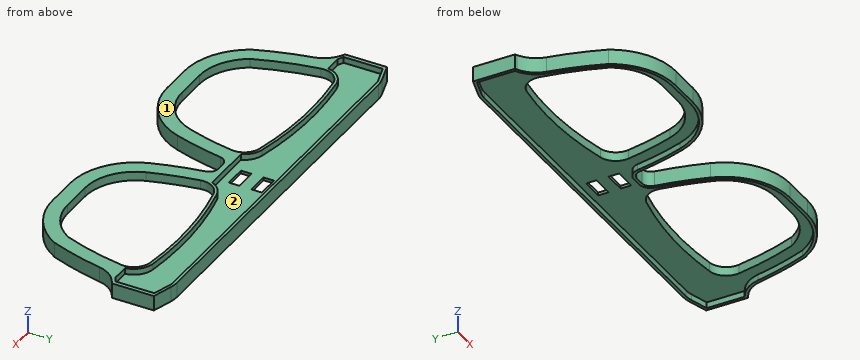
from build123d import *

# Parameters (mm, degrees)
BOSS_EXTRUDE1_DEPTH  = 5
CUT_EXTRUDE1_DEPTH   = 78.98076686
FILLET1_R            = 6
FILLET4_R            = 3
FILLET5_R            = 10
FILLET1_OF_MIRROR2_R = 6
FILLET4_OF_MIRROR2_R = 3
FILLET5_OF_MIRROR2_R = 10
CUT_EXTRUDE2_DEPTH   = 2
SKETCH4_W            = 7.3
SKETCH4_H            = 3.5
CUT_EXTRUDE3_DEPTH   = 78.878110027
CUT_EXTRUDE4_START   = -1
CUT_EXTRUDE4_DEPTH   = 2


with BuildPart() as part:
    # Sketch1 → Boss-Extrude1 (new body)
    with BuildSketch(Plane.XY):
        with BuildLine():
            Line((-70, 16.58258549), (-70, 2.58258549))
            Line((-70, 2.58258549), (-65, -0.035347018))
            ThreePointArc((-65, -0.035347018), (-62.639321295, -11.428715409), (-59.057390955, -22.499009997))
            ThreePointArc((-59.057390955, -22.499009997), (-50.858075368, -30.911196539), (-39.524366721, -34))
            Line((-39.524366721, -34), (-29.119439011, -34))
            ThreePointArc((-29.119439011, -34), (-16.364659062, -29.873537236), (-8.443933007, -19.058075838))
            ThreePointArc((-8.443933007, -19.058075838), (-5.792248942, -9.629238804), (-4, 0))
            Line((-4, 0), (0, 0))
            Line((0, 0), (0, 19))
            Line((0, 19), (-62, 19))
            Line((-62, 19), (-70, 16.58258549))
        make_face()
    boss_extrude1 = extrude(amount=BOSS_EXTRUDE1_DEPTH)

    # Sketch2 → Cut-Extrude1 (cut, through all)
    with BuildSketch(Plane.XY.offset(5)):
        with BuildLine():
            Line((-39.524366721, -29), (-29.119439011, -29))
            ThreePointArc((-29.119439011, -29), (-19.293350153, -25.821035725), (-13.191343035, -17.488968441))
            ThreePointArc((-13.191343035, -17.488968441), (-10.661621804, -8.493805879), (-8.951806424, 0.692541077))
            ThreePointArc((-8.951806424, 0.692541077), (-8.83111114, 2.375291538), (-8.93749946, 4.05900707))
            ThreePointArc((-8.93749946, 4.05900707), (-33.987475013, 7.999161751), (-59.288689209, 6.303681198))
            ThreePointArc((-59.288689209, 6.303681198), (-60.075532666, 3.563074376), (-60.056140486, 0.711816353))
            ThreePointArc((-60.056140486, 0.711816353), (-57.852345066, -9.972645379), (-54.521869403, -20.361214511))
            ThreePointArc((-54.521869403, -20.361214511), (-48.178176596, -26.685865227), (-39.524366721, -29))
        make_face()
    cut_extrude1 = extrude(amount=-CUT_EXTRUDE1_DEPTH, mode=Mode.SUBTRACT)

    # Fillet1
    fillet1_edges = [part.edges().sort_by_distance(p)[0] for p in [
        (-8.93749946, 4.05900707, 2.5),
        (-59.288689209, 6.303681198, 2.5),
    ]]
    fillet(fillet1_edges, radius=FILLET1_R)

    # Fillet4
    fillet4_edges = [part.edges().sort_by_distance(p)[0] for p in [
        (-4, 0, 2.5),
    ]]
    fillet(fillet4_edges, radius=FILLET4_R)

    # Fillet5
    fillet5_edges = [part.edges().sort_by_distance(p)[0] for p in [
        (-65, -0.035347018, 2.5),
        (-62, 19, 2.5),
    ]]
    fillet(fillet5_edges, radius=FILLET5_R)

    # Mirror2: Boss-Extrude1, Cut-Extrude1 across plane
    add(boss_extrude1.mirror(Plane(origin=(0, 19, 5), x_dir=(0, 0, 1), z_dir=(1, 0, 0))))
    add(cut_extrude1.mirror(Plane(origin=(0, 19, 5), x_dir=(0, 0, 1), z_dir=(1, 0, 0))), mode=Mode.SUBTRACT)

    # Fillet1 of Mirror2
    fillet1_of_mirror2_edges = [part.edges().sort_by_distance(p)[0] for p in [
        (8.93749946, 4.05900707, 2.5),
        (59.288689209, 6.303681198, 2.5),
    ]]
    fillet(fillet1_of_mirror2_edges, radius=FILLET1_OF_MIRROR2_R)

    # Fillet4 of Mirror2
    fillet4_of_mirror2_edges = [part.edges().sort_by_distance(p)[0] for p in [
        (4, 0, 2.5),
    ]]
    fillet(fillet4_of_mirror2_edges, radius=FILLET4_OF_MIRROR2_R)

    # Fillet5 of Mirror2
    fillet5_of_mirror2_edges = [part.edges().sort_by_distance(p)[0] for p in [
        (65, -0.035347018, 2.5),
        (62, 19, 2.5),
    ]]
    fillet(fillet5_of_mirror2_edges, radius=FILLET5_OF_MIRROR2_R)

    # Sketch3 → Cut-Extrude2 (cut)
    with BuildSketch(Plane.XY.offset(5)):
        with BuildLine():
            Line((-61.852211578, 18), (-68.579000582, 15.967320332))
            Line((-68.579000582, 15.967320332), (-68.579000582, 2.967348727))
            Line((-68.579000582, 2.967348727), (-66.731457293, 2))
            Line((-66.731457293, 2), (-60.978148267, 2))
            ThreePointArc((-60.978148267, 2), (-59.004204322, 6.004331826), (-55.011184694, 8.001059729))
            ThreePointArc((-55.011184694, 8.001059729), (-34.257732376, 9.011771002), (-13.66121584, 6.271182212))
            ThreePointArc((-13.66121584, 6.271182212), (-10.64537641, 4.753154175), (-8.690935653, 2))
            Line((-8.690935653, 2), (-4.382114171, 2))
            Line((-4.382114171, 2), (0, 2))
            Line((0, 2), (0, 18))
            Line((0, 18), (-61.852211578, 18))
        make_face()
        with BuildLine():
            Line((61.852211578, 18), (0, 18))
            Line((0, 18), (0, 2))
            Line((0, 2), (4.382114171, 2))
            Line((4.382114171, 2), (8.690935653, 2))
            ThreePointArc((8.690935653, 2), (10.64537641, 4.753154175), (13.66121584, 6.271182212))
            ThreePointArc((13.66121584, 6.271182212), (34.257732376, 9.011771002), (55.011184694, 8.001059729))
            ThreePointArc((55.011184694, 8.001059729), (59.004204322, 6.004331826), (60.978148267, 2))
            Line((60.978148267, 2), (66.731457293, 2))
            Line((66.731457293, 2), (68.579000582, 2.967348727))
            Line((68.579000582, 2.967348727), (68.579000582, 15.967320332))
            Line((68.579000582, 15.967320332), (61.852211578, 18))
        make_face()
    extrude(amount=-CUT_EXTRUDE2_DEPTH, mode=Mode.SUBTRACT)

    # Sketch4 → Cut-Extrude3 (cut, through all)
    with BuildSketch(Plane.XY.offset(3)):
        with Locations((0, 14)):
            Rectangle(SKETCH4_W, SKETCH4_H)
        with Locations((0, 6.5)):
            Rectangle(SKETCH4_W, SKETCH4_H)
    extrude(amount=-CUT_EXTRUDE3_DEPTH, mode=Mode.SUBTRACT)

    # Sketch6 → Cut-Extrude4 (cut)
    with BuildSketch(Plane.XY.offset(3).offset(CUT_EXTRUDE4_START)):
        with BuildLine():
            Line((69, 15.840104069), (63.125446932, 17.615257798))
            ThreePointArc((63.125446932, 17.615257798), (61.837919684, 17.903294901), (60.522115781, 18))
            Line((60.522115781, 18), (-60.522115781, 18))
            ThreePointArc((-60.522115781, 18), (-61.837919684, 17.903294901), (-63.125446932, 17.615257798))
            Line((-63.125446932, 17.615257798), (-69, 15.840104069))
            Line((-69, 15.840104069), (-69, 3.18777834))
            Line((-69, 3.18777834), (-68.903213495, 3.137102232))
            ThreePointArc((-68.903213495, 3.137102232), (-65.190574761, -0.027998941), (-63.211910581, -4.487420414))
            ThreePointArc((-63.211910581, -4.487420414), (-61.060268821, -13.390129723), (-58.149320801, -22.074263356))
            ThreePointArc((-58.149320801, -22.074263356), (-50.3209013, -30.066984302), (-39.524366721, -33))
            Line((-39.524366721, -33), (-29.119439011, -33))
            ThreePointArc((-29.119439011, -33), (-16.95039728, -29.063036934), (-9.393415013, -18.744254359))
            ThreePointArc((-9.393415013, -18.744254359), (-7.059487639, -10.627794467), (-5.368651351, -2.353423746))
            ThreePointArc((-5.368651351, -2.353423746), (-4.01101304, 0.048467239), (-1.421254848, 1))
            Line((-1.421254848, 1), (1.421254848, 1))
            ThreePointArc((1.421254848, 1), (4.01101304, 0.048467239), (5.368651351, -2.353423746))
            ThreePointArc((5.368651351, -2.353423746), (7.059487639, -10.627794467), (9.393415013, -18.744254359))
            ThreePointArc((9.393415013, -18.744254359), (16.95039728, -29.063036934), (29.119439011, -33))
            Line((29.119439011, -33), (39.524366721, -33))
            ThreePointArc((39.524366721, -33), (50.3209013, -30.066984302), (58.149320801, -22.074263356))
            ThreePointArc((58.149320801, -22.074263356), (61.060268821, -13.390129723), (63.211910581, -4.487420414))
            ThreePointArc((63.211910581, -4.487420414), (65.190574761, -0.027998941), (68.903213495, 3.137102232))
            Line((68.903213495, 3.137102232), (69, 3.18777834))
            Line((69, 3.18777834), (69, 15.840104069))
        make_face()
        with BuildLine():
            Line((39.524366721, -29), (29.119439011, -29))
            ThreePointArc((29.119439011, -29), (19.293350153, -25.821035725), (13.191343035, -17.488968441))
            ThreePointArc((13.191343035, -17.488968441), (10.920912078, -9.579342567), (9.284744219, -1.514604944))
            ThreePointArc((9.284744219, -1.514604944), (10.234661813, 2.801128318), (13.882135009, 5.295890091))
            ThreePointArc((13.882135009, 5.295890091), (34.299530853, 8.01264494), (54.872497662, 7.010723469))
            ThreePointArc((54.872497662, 7.010723469), (58.860128117, 4.642217415), (59.967820133, 0.138437228))
            ThreePointArc((59.967820133, 0.138437228), (57.77826599, -10.253097668), (54.521869403, -20.361214511))
            ThreePointArc((54.521869403, -20.361214511), (48.178176596, -26.685865227), (39.524366721, -29))
        make_face(mode=Mode.SUBTRACT)
        with BuildLine():
            Line((-39.524366721, -29), (-29.119439011, -29))
            ThreePointArc((-29.119439011, -29), (-19.293350153, -25.821035725), (-13.191343035, -17.488968441))
            ThreePointArc((-13.191343035, -17.488968441), (-10.920912078, -9.579342567), (-9.284744219, -1.514604944))
            ThreePointArc((-9.284744219, -1.514604944), (-10.234661813, 2.801128318), (-13.882135009, 5.295890091))
            ThreePointArc((-13.882135009, 5.295890091), (-34.299530853, 8.01264494), (-54.872497662, 7.010723469))
            ThreePointArc((-54.872497662, 7.010723469), (-58.860128117, 4.642217415), (-59.967820133, 0.138437228))
            ThreePointArc((-59.967820133, 0.138437228), (-57.77826599, -10.253097668), (-54.521869403, -20.361214511))
            ThreePointArc((-54.521869403, -20.361214511), (-48.178176596, -26.685865227), (-39.524366721, -29))
        make_face(mode=Mode.SUBTRACT)
    extrude(amount=-CUT_EXTRUDE4_DEPTH, mode=Mode.SUBTRACT)


solid = part.part
Build history of the part. All positions in model axes, mm. Face numbers are marked on the shaded views. Give positions to 0.01 mm unless a question says otherwise; leave off trailing zeros. Order: outer loops, then holes, each group sorted by start corner. A loop starts at its lowest first (then second) coordinate and runs counter-clockwise, first axis right, second up. Notation, with made-up numbers: M 26,28.25 L 46,28.25 A22 ccw 46,52.25 Z; hole C -10,-18.75 d11. An arc over 180 degrees is marked long. Use one line per item in the form item = value.
1) Saw through at A-A (y = 14). Give the cut face in (x, z).
Calculated:
outline = M -70,0 L -69,0 L -69,2 L -3.65,2 L -3.65,3 L -68.58,3 L -68.58,5 L -70,5 Z; M 3.65,2 L 69,2 L 69,0 L 70,0 L 70,5 L 68.58,5 L 68.58,3 L 3.65,3 Z
2) Probe probe 1 along X at (y, z) = (12, 3.85); probe 2 along X at (y, z) = (-27.5, 2.8); probe 3 along X at (y, z) = (-18.5, 0.7). List the from-to ranges inside material, lowest first.
Calculated:
probe_1 = -70 to -68.58, 68.58 to 70
probe_2 = -55.28 to -46.58, -22.19 to -13.6, 13.6 to 22.19, 46.58 to 55.28
probe_3 = -60.51 to -59.45, -9.31 to -8.26, 8.26 to 9.31, 59.45 to 60.51
3) Saw through at C-C (y = -15.5). Give the cut face in (x, z).
Calculated:
outline = M -61.48,0 L -60.43,0 L -60.43,2 L -56.23,2 L -56.23,5 L -61.48,5 Z; M -12.56,2 L -8.38,2 L -8.38,0 L -7.34,0 L -7.34,5 L -12.56,5 Z; M 7.34,0 L 8.38,0 L 8.38,2 L 12.56,2 L 12.56,5 L 7.34,5 Z; M 56.23,2 L 60.43,2 L 60.43,0 L 61.48,0 L 61.48,5 L 56.23,5 Z
4) Saw through at B-B (x = -24.5). Give the cut face in (y, z), plus the area to 3 significant figures.
Calculated:
outline = M -33.5,0 L -32.48,0 L -32.48,2 L -28.35,2 L -28.35,5 L -33.5,5 Z; M 7.18,2 L 18,2 L 18,0 L 19,0 L 19,5 L 18,5 L 18,3 L 8.19,3 L 8.19,5 L 7.18,5 Z
area = 35.3 mm2
5) Two-plate mould, pull along Y, no slides. Class the marked faces 1 and 2: released by +Y, released by -Y, zero draft, split by the parting line, or undercut.
Calculated:
face_1 = zero draft
face_2 = undercut
6) Saw through at D-D (z = 4). State how many separate pieces and enclosed holes the cut face has, plus the area to 3 significant figures.
Calculated:
separate_pieces = 1
enclosed_holes = 3
area = 1,330 mm2
7) Drop flat-ended pins along their axis: pin 1 (2 mm diameter, centred on x = -64, z = 4.5, fed in from +Y); pin 2 (3 mm diameter, centred on x = -0.5, z = 3, fed in from -Y); pin 3 (2 mm diameter, centred on x = 15.5, z = 4.5, fed in from -Y). Give the stop position or say it passes through.
Calculated:
pin_1 = 18.69
pin_2 = -0.06
pin_3 = -29.97
